Can you work these out from the model? Positions are in its coordinate system, mm. A direction names the side the tool comes from. Coordinates: 2 decimals unless noted, no trailing zeros. Loops run counter-clockwise (first coordinate to the right, second up) from the corner with the lowest first, then second, coordinate; pieces in that order, holes last. Notation, with made-up numbers: (20.5, 0) -> (49.5, 0) arc R23 cw to (49.5, 30) -> close; hole circle Ø9 at (25.5, 70.25). An arc over 180 degrees is marked (long way). Use one line per item in the form item = value. Start each with the question number.
(1) I'm going to push flat-ended pins straight in: pin 1 (1.5 mm diameter, centred on x = -9, y = 32, fed in from -Z); pin 2 (7 mm diameter, centred on x = -17, y = 21, fed in from +Z); pin 3 (1.4 mm diameter, centred on x = -19.5, y = 34, fed in from +Z). Where does each tip first touch, or does it pass through?
(2) Imagine slicing it at C-C (x = -7.5). List the corners of the cut face in (y, z) for me, plus the area to 3 significant figures.
(3) I need wall thicknesses on line 1 (X direction, y = 36, z = -37); line 2 (Y direction, x = -14.75, z = -63); line 3 (Z direction, x = -15.5, y = 36.5). Which ranges of each line are inside material? Lowest first, please. Write a range as [from, to].
(4) Imagine slicing it at D-D (y = 11). List the corners of the cut face in (x, z) for me, plus the area to 3 significant figures.
(5) On a 3-axis mill with a long thin cutter (end or side, diameter ignored), from which of +Z, -Z, +X, -X, +Y, -Y can I reach the whole of each face in a straight line? I mean faces 1 (the flat face through (-12, 10, -26)), 2 (the flat face through (-11, 34, -38)), 3 (the flat face through (-19, 34, -40.35)). Say none if no direction works.
(6) Imagine slicing it at A-A (z = -37.5). List the corners of the cut face in (x, y) for me, plus the area to 3 significant figures.
(7) Imagine slicing it at B-B (z = -63). List the corners of the cut face in (x, y) for me.
(8) Thinking about a two-plate mould opening in Z: for faces 4 (the flat face through (-5, 32.8, -38)), 5 (the cylindrical face through (-11.83, 23.99, -72.15)), 6 (the flat face through (0, 15, -37)), which applies, released by +Z, released by -Z, zero draft, split by the parting line, or undercut?
```python
from build123d import *

# Parameters (mm, degrees)
SKETCH1_W           = 24
SKETCH1_H           = 75
BOSS_EXTRUDE1_DEPTH = 10
SKETCH2_W           = 24
SKETCH2_H           = 24
BOSS_EXTRUDE2_DEPTH = 17
SKETCH3_R           = 7.5
CUT_EXTRUDE1_DEPTH  = 25
FILLET1_R           = 10
SKETCH4_W           = 24
SKETCH4_H           = 19
BOSS_EXTRUDE3_DEPTH = 28.5
SKETCH5_W           = 5.7
SKETCH5_H           = 2.7
CUT_EXTRUDE2_DEPTH  = 11
CUT_EXTRUDE3_START  = -24
SKETCH5_2_W         = 5.7
SKETCH5_2_H         = 2.7
CUT_EXTRUDE3_DEPTH  = 11
CUT_EXTRUDE4_REACH  = 40.5
SKETCH6_R           = 1.65


with BuildPart() as part:
    # Sketch1 → Boss-Extrude1 (new body)
    with BuildSketch(Plane(origin=(0, 0, 0), x_dir=(1, 0, 0), z_dir=(0, 1, 0))):
        with Locations((-12, 37.5)):
            Rectangle(SKETCH1_W, SKETCH1_H)
    extrude(amount=BOSS_EXTRUDE1_DEPTH)

    # Sketch2 → Boss-Extrude2 (add)
    with BuildSketch(Plane(origin=(0, 10, 0), x_dir=(1, 0, 0), z_dir=(0, 1, 0))):
        with Locations((-12, 12)):
            Rectangle(SKETCH2_W, SKETCH2_H)
        with Locations((-12, 63)):
            Rectangle(SKETCH2_W, SKETCH2_H)
    extrude(amount=BOSS_EXTRUDE2_DEPTH)

    # Sketch3 → Cut-Extrude1 (cut, through all)
    with BuildSketch(Plane(origin=(0, 0, 0), x_dir=(0, 0, -1), z_dir=(1, 0, 0))):
        with Locations((12, 17.5)):
            Circle(SKETCH3_R)
        with Locations((63, 17.5)):
            Circle(SKETCH3_R)
    extrude(amount=-CUT_EXTRUDE1_DEPTH, mode=Mode.SUBTRACT)

    # Fillet1
    fillet1_edges = [part.edges().sort_by_distance(p)[0] for p in [
        (-12, 27, -51),
        (-12, 27, -24),
        (-12, 27, 0),
        (-12, 27, -75),
    ]]
    fillet(fillet1_edges, radius=FILLET1_R)

    # Sketch4 → Boss-Extrude3 (add)
    with BuildSketch(Plane(origin=(0, 10, 0), x_dir=(1, 0, 0), z_dir=(0, 1, 0))):
        with Locations((-12, 37.5)):
            Rectangle(SKETCH4_W, SKETCH4_H)
    extrude(amount=BOSS_EXTRUDE3_DEPTH)

    # Sketch5 → Cut-Extrude2 (cut)
    with BuildSketch(Plane.ZY.offset(24)):
        with Locations((-37.5, 34.15)):
            Rectangle(SKETCH5_W, SKETCH5_H)
    extrude(amount=-CUT_EXTRUDE2_DEPTH, mode=Mode.SUBTRACT)

    # Sketch5<2> → Cut-Extrude3 (cut)
    with BuildSketch(Plane.ZY.offset(24).offset(CUT_EXTRUDE3_START)):
        with Locations((-37.5, 34.15)):
            Rectangle(SKETCH5_2_W, SKETCH5_2_H)
    extrude(amount=CUT_EXTRUDE3_DEPTH, mode=Mode.SUBTRACT)

    # Sketch6 → Cut-Extrude4 (cut, up to next)
    with BuildSketch(Plane(origin=(0, 38.5, 0), x_dir=(1, 0, 0), z_dir=(0, 1, 0)), mode=Mode.PRIVATE) as cut_extrude4_sk1:
        with Locations((-4.65, 37.5)):
            Circle(SKETCH6_R)
    cut_extrude4_tool1 = extrude(cut_extrude4_sk1.sketch, amount=-CUT_EXTRUDE4_REACH, mode=Mode.PRIVATE) & part.part
    add(cut_extrude4_tool1.solids().sort_by_distance((-4.65, 38.5, -37.5))[0], mode=Mode.SUBTRACT)
    # Sketch6 → Cut-Extrude4 (cut, up to next)
    with BuildSketch(Plane(origin=(0, 38.5, 0), x_dir=(1, 0, 0), z_dir=(0, 1, 0)), mode=Mode.PRIVATE) as cut_extrude4_sk2:
        with Locations((-19.35, 37.5)):
            Circle(SKETCH6_R)
    cut_extrude4_tool2 = extrude(cut_extrude4_sk2.sketch, amount=-CUT_EXTRUDE4_REACH, mode=Mode.PRIVATE) & part.part
    add(cut_extrude4_tool2.solids().sort_by_distance((-19.35, 38.5, -37.5))[0], mode=Mode.SUBTRACT)


solid = part.part
```
Worked out:
q1.pin_1 = -47
q1.pin_2 = -0.01
q1.pin_3 = -28
q2.outline = (0, -75) -> (17, -75) arc R10 ccw to (27, -65) -> (27, -61) arc R10 ccw to (17, -51) -> (10, -51) -> (10, -47) -> (38.5, -47) -> (38.5, -28) -> (10, -28) -> (10, -24) -> (17, -24) arc R10 ccw to (27, -14) -> (27, -10) arc R10 ccw to (17, 0) -> (0, 0) -> close; hole circle Ø15 at (17.5, -63); hole circle Ø15 at (17.5, -12); hole (32.8, -40.35) -> (35.5, -40.35) -> (35.5, -34.65) -> (32.8, -34.65) -> close
q2.area = 1,650 mm2
q3.line_1 = [-24, -20.92], [-17.78, -6.22], [-3.08, 0]
q3.line_2 = [0, 10], [25, 27]
q3.line_3 = [-47, -28]
q4.outline = (-24, -75) -> (0, -75) -> (0, -66.74) -> (-24, -66.74) -> close; (-24, -59.26) -> (0, -59.26) -> (0, -51) -> (-24, -51) -> close; (-24, -47) -> (0, -47) -> (0, -28) -> (-24, -28) -> close; (-24, -24) -> (0, -24) -> (0, -15.74) -> (-24, -15.74) -> close; (-24, -8.26) -> (0, -8.26) -> (0, 0) -> (-24, 0) -> close
q4.area = 1,250 mm2
q5.face_1 = +X, -X, +Y
q5.face_2 = +X
q5.face_3 = -X
q6.outline = (-24, 0) -> (0, 0) -> (0, 32.8) -> (-11, 32.8) -> (-11, 35.5) -> (-6.3, 35.5) -> (-6.3, 38.5) -> (-17.7, 38.5) -> (-17.7, 35.5) -> (-13, 35.5) -> (-13, 32.8) -> (-24, 32.8) -> close; (-24, 35.5) -> (-21, 35.5) -> (-21, 38.5) -> (-24, 38.5) -> close; (-3, 35.5) -> (0, 35.5) -> (0, 38.5) -> (-3, 38.5) -> close
q6.area = 845 mm2
q7.outline = (-24, 0) -> (0, 0) -> (0, 10) -> (-24, 10) -> close; (-24, 25) -> (0, 25) -> (0, 27) -> (-24, 27) -> close
q8.face_4 = undercut
q8.face_5 = released by -Z
q8.face_6 = zero draft
